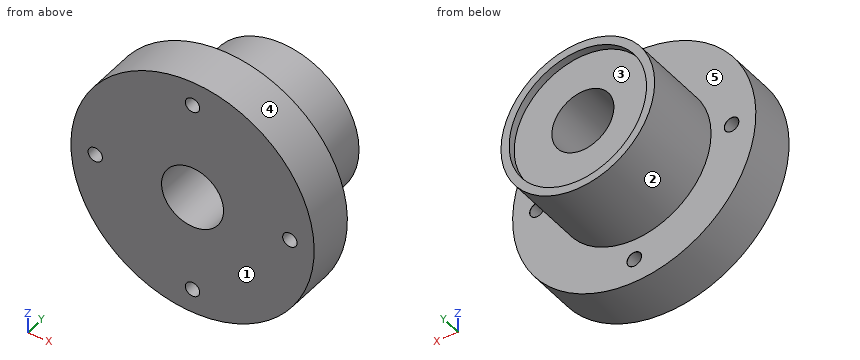
```python
from build123d import *

# Parameters (mm, degrees)
SKETCH1_R                       = 25.4
BOSS_EXTRUDE1_DEPTH             = 25.4
SKETCH2_OUTSIDE_W               = 68.04
SKETCH2_OUTSIDE_H               = 68.04
SKETCH2_OUTSIDE_R               = 16.05
CUT_EXTRUDE1_DEPTH              = 15.422
SKETCH3_R                       = 6.477
CUT_EXTRUDE2_DEPTH              = 44.994090512
BOSS_EXTRUDE2_START             = 1.524
SKETCH4_R                       = 16.05
SKETCH4_R_2                     = 14.351
BOSS_EXTRUDE2_DEPTH             = 1.524
F_3_0MM_DOWEL_HOLE1_D           = 3
F_3_0MM_DOWEL_HOLE1_CSINK_D     = 3.05
F_3_0MM_DOWEL_HOLE1_CSINK_ANGLE = 90
CIRPATTERN1_COUNT               = 4


with BuildPart() as part:
    # Sketch1 → Boss-Extrude1 (new body)
    with BuildSketch(Plane(origin=(0, 0, 0), x_dir=(1, 0, 0), z_dir=(0, 1, 0))):
        with Locations(Location((0, 0, 0), (0, 0, 270))):
            Circle(SKETCH1_R)
    extrude(amount=BOSS_EXTRUDE1_DEPTH)

    # Sketch2 outside → Cut-Extrude1 (cut)
    with BuildSketch(Plane(origin=(0, 25.4, 0), x_dir=(1, 0, 0), z_dir=(0, 1, 0))):
        Rectangle(SKETCH2_OUTSIDE_W, SKETCH2_OUTSIDE_H)
        with Locations(Location((0, 0, 0), (0, 0, 270))):
            Circle(SKETCH2_OUTSIDE_R, mode=Mode.SUBTRACT)
    extrude(amount=-CUT_EXTRUDE1_DEPTH, mode=Mode.SUBTRACT)

    # Sketch3 → Cut-Extrude2 (cut, through all)
    with BuildSketch(Plane.XZ):
        with Locations(Location((0, 0, 0), (0, 0, 270))):
            Circle(SKETCH3_R)
    extrude(amount=-CUT_EXTRUDE2_DEPTH, mode=Mode.SUBTRACT)

    # Sketch4 → Boss-Extrude2 (add)
    with BuildSketch(Plane(origin=(0, 25.4, 0), x_dir=(1, 0, 0), z_dir=(0, 1, 0)).offset(BOSS_EXTRUDE2_START)):
        with Locations(Location((0, 0, 0), (0, 0, 270))):
            Circle(SKETCH4_R)
        with Locations(Location((0, 0, 0), (0, 0, 90))):
            Circle(SKETCH4_R_2, mode=Mode.SUBTRACT)
    extrude(amount=-BOSS_EXTRUDE2_DEPTH)

    # Ø3.0mm Dowel Hole1 (through all)
    with Locations(Plane(origin=(0, 9.978, -20.32), x_dir=(0, 0, 1), z_dir=(0, 1, 0))):
        with Locations((0, 0)):
            f_3_0mm_dowel_hole1 = CounterSinkHole(F_3_0MM_DOWEL_HOLE1_D / 2, F_3_0MM_DOWEL_HOLE1_CSINK_D / 2, counter_sink_angle=F_3_0MM_DOWEL_HOLE1_CSINK_ANGLE)

    # CirPattern1: Ø3.0mm Dowel Hole1 ×4 about axis
    cirpattern1_axis = Axis((0, 0, 0), (0, 1, 0))
    for i in range(1, CIRPATTERN1_COUNT):
        add(f_3_0mm_dowel_hole1.rotate(cirpattern1_axis, i * 360 / CIRPATTERN1_COUNT), mode=Mode.SUBTRACT)


solid = part.part
```
Geometry: final body of the model. Coordinates: model frame, mm. Face numbers are marked on the shaded views. A direction names the side the tool comes from. Coordinates: 2 decimals unless noted, no trailing zeros. Order: outer loops, then holes, each group sorted by start corner. A loop starts at its lowest first (then second) coordinate and runs counter-clockwise, first axis right, second up.
Item 1: Draft query along Z for the marked faces 3, 4 and 5. Return one class per face: released by +Z, released by -Z, zero draft, split by the parting line, or undercut.
Answer:
face 3: undercut
face 4: split by the parting line
face 5: zero draft
Item 2: Contact query for flat-ended pins moving along their axis: P1, Ø12, axis at x = -3.5, y = 5, coming from the +Z side; P2, Ø3, axis at x = 20, z = 12, coming from the +Y side; P3, Ø6, axis at y = 6, z = 3.5, coming from the +X side; P4, Ø6, axis at x = -16.5, y = 23, coming from the -Z side. Output: stop coordinate, or through.
Answer:
P1: stops at z = 25.4
P2: stops at y = 9.98
P3: stops at x = 25.4
P4: stops at z = -8.68
Item 3: Section query D-D (y = 8.5). Output: boundary loops of the cut face in (x, z), then the cut area to 3 significant figures.
Answer:
outline: circle Ø50.8 at (0, 0); hole circle Ø3 at (-20.32, 0); hole circle Ø12.95 at (0, 0); hole circle Ø3 at (0, -20.32); hole circle Ø3 at (0, 20.32); hole circle Ø3 at (20.32, 0)
area: 1,870 mm2
Item 4: Section query A-A (z = 0). Output: boundary loops of the cut face in (x, y) (3 decimals), then the cut area to 3 significant figures.
Answer:
outline: (-25.4, 0) - (-21.82, 0) - (-21.82, 9.953) - (-21.845, 9.978) - (-25.4, 9.978) - close; (-18.82, 0) - (-6.477, 0) - (-6.477, 25.4) - (-14.351, 25.4) - (-14.351, 26.924) - (-16.05, 26.924) - (-16.05, 9.978) - (-18.795, 9.978) - (-18.82, 9.953) - close; (6.477, 0) - (18.82, 0) - (18.82, 9.953) - (18.795, 9.978) - (16.05, 9.978) - (16.05, 26.924) - (14.351, 26.924) - (14.351, 25.4) - (6.477, 25.4) - close; (21.82, 0) - (25.4, 0) - (25.4, 9.978) - (21.845, 9.978) - (21.82, 9.953) - close
area: 618 mm2
Item 5: Section query B-B (x = 0). Output: boundary loops of the cut face in (y, z) (3 decimals), then the cut area to 3 significant figures.
Answer:
outline: (0, -25.4) - (9.978, -25.4) - (9.978, -21.845) - (9.953, -21.82) - (0, -21.82) - close; (0, -18.82) - (9.953, -18.82) - (9.978, -18.795) - (9.978, -16.05) - (26.924, -16.05) - (26.924, -14.351) - (25.4, -14.351) - (25.4, -6.477) - (0, -6.477) - close; (0, 6.477) - (25.4, 6.477) - (25.4, 14.351) - (26.924, 14.351) - (26.924, 16.05) - (9.978, 16.05) - (9.978, 18.795) - (9.953, 18.82) - (0, 18.82) - close; (0, 21.82) - (9.953, 21.82) - (9.978, 21.845) - (9.978, 25.4) - (0, 25.4) - close
area: 618 mm2
Item 6: Material intervals for line 1 along X through (y, z) = (26.3, 0); line 2 along Y through (x, z) = (-0.5, 6.5); line 3 along X through (y, z) = (12, 0), sorted ascending.
Answer:
line 1: x = -16.05 to -14.35, 14.35 to 16.05
line 2: y = 0 to 25.4
line 3: x = -16.05 to -6.48, 6.48 to 16.05
Item 7: Section query C-C (x = -20.32). Output: boundary loops of the cut face in (y, z) (3 decimals).
Answer:
outline: (0, -15.24) - (9.978, -15.24) - (9.978, -1.525) - (9.953, -1.5) - (0, -1.5) - close; (0, 1.5) - (9.953, 1.5) - (9.978, 1.525) - (9.978, 15.24) - (0, 15.24) - close
Item 8: Access query for the marked faces 1 and 2. Directions: +Z, -Z, +X, -X, +Y, -Y. A direction counts if a zero-diameter tool reaches every point of the face in a straight line with its end or side. Return the directions, or none.
Answer:
face 1: +Z, -Z, +X, -X, -Y
face 2: +Y
